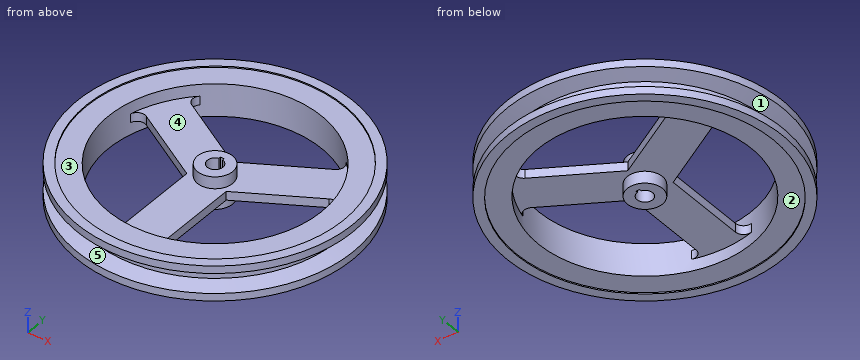
```python
from build123d import *

# Parameters (mm, degrees)
EXTRUDE_1_DEPTH     = 3.5
FILLET_1_R          = 6.5
SKETCH_4_R          = 14
EXTRUDE_2_DEPTH     = 13
CUT_EXTRUDE_1_DEPTH = 13


with BuildPart() as part:
    # 草图2 → 旋转1 (revolve)
    with BuildSketch(Plane(origin=(0, 0, 0), x_dir=(0, 0, -1), z_dir=(1, 0, 0)), mode=Mode.PRIVATE) as revolve_1_sk:
        Polygon((14, 102.5), (14, 110), (8, 110), (5.707749251, 97), (-5.707749251, 97), (-8, 110), (-14, 110), (-14, 102.5), (-13, 102.5), (-13, 85), (13, 85), (13, 102.5), align=None)
    revolve(revolve_1_sk.sketch.rotate(Axis((0, 0, 67.916666667), (0, 0, -1)), 90), axis=Axis((0, 0, 67.916666667), (0, 0, -1)))

    # 草图3 → 凸台-拉伸1 (add, symmetric)
    with BuildSketch(Plane.XY):
        with BuildLine():
            Line((0, 18.186533479), (-64.462425479, 55.403932183))
            ThreePointArc((-64.462425479, 55.403932183), (-73.612159322, 42.5), (-80.212425479, 28.124131963))
            Line((-80.212425479, 28.124131963), (-15.75, -9.09326674))
            Line((-15.75, -9.09326674), (-15.75, -83.528064146))
            ThreePointArc((-15.75, -83.528064146), (0, -85), (15.75, -83.528064146))
            Line((15.75, -83.528064146), (15.75, -9.09326674))
            Line((15.75, -9.09326674), (80.212425479, 28.124131963))
            ThreePointArc((80.212425479, 28.124131963), (73.612159322, 42.5), (64.462425479, 55.403932183))
            Line((64.462425479, 55.403932183), (0, 18.186533479))
        make_face()
    extrude(amount=EXTRUDE_1_DEPTH, both=True)

    # 圆角1
    fillet_1_edges = [part.edges().sort_by_distance(p)[0] for p in [
        (64.462425479, 55.403932183, 0),
        (-64.462425479, 55.403932183, 0),
        (-80.212425479, 28.124131963, 0),
        (-15.75, -83.528064146, 0),
        (15.75, -83.528064146, 0),
        (80.212425479, 28.124131963, 0),
    ]]
    fillet(fillet_1_edges, radius=FILLET_1_R)

    # 草图4 → 凸台-拉伸2 (add, symmetric)
    with BuildSketch(Plane.XY):
        with Locations(Location((0, 0, 0), (0, 0, 180))):
            Circle(SKETCH_4_R)
    extrude(amount=EXTRUDE_2_DEPTH, both=True)

    # 草图5 → 切除-拉伸1 (cut, symmetric)
    with BuildSketch(Plane.XY):
        with BuildLine():
            Line((-1.5, 6.06733055), (-1.5, 7.75))
            Line((-1.5, 7.75), (1.5, 7.75))
            Line((1.5, 7.75), (1.5, 6.06733055))
            ThreePointArc((1.5, 6.06733055), (0, -6.25), (-1.5, 6.06733055))
        make_face()
    extrude(amount=CUT_EXTRUDE_1_DEPTH, both=True, mode=Mode.SUBTRACT)


solid = part.part
```
Model file for the job. Use its own axes, mm. Face numbers are marked on the shaded views. A direction names the side the tool comes from. Round coordinates to 2 decimals unless told otherwise and drop trailing zeros. Put each result on its own line as item: value. Start each with the question number.
Item 1: Drill centre lines: line 1 along Y through (x, z) = (18.5, 0.75); line 2 along X through (y, z) = (3, 11); line 3 along Y through (x, z) = (0, -13.6). Where is each one in solid material? Low to high.
Item 2: Mould opens along Y. For the marked faces 4 and 5 say: released by +Y, released by -Y, zero draft, split by the parting line, or undercut.
Item 3: 3-axis set-ups, long thin cutter, end or side, ignore diameter. For the marked faces 1, 2 and 3: which of +Z, -Z, +X, -X, +Y, -Y reach the whole face in a straight line?
Item 4: Cut at A-A (y = 0). Give the number of separate pieces and of enclosed holes in the cut face, then the cut area to 3 significant figures.
Item 5: Drop flat-ended pins along their axis: P1, Ø10, axis at x = -53, y = 18.5, coming from the +Z side; P2, Ø14, axis at x = -6.5, y = 2, coming from the +Z side; P3, Ø12, axis at x = 81, z = 3, coming from the -Y side; P4, Ø8, axis at x = -83, y = -79, coming from the +Z side. Give the stop position or say it passes through.
Answer block:
1. line 1: -95.22 to -80.59, -7.51 to 28.87, 82.96 to 95.22
1. line 2: -109.96 to -84.95, -13.67 to -5.48, 5.48 to 13.67, 84.95 to 109.96
1. line 3: -110 to -102.5, 102.5 to 110
2. face 4: undercut
2. face 5: split by the parting line
3. face 1: none
3. face 2: -Z
3. face 3: +Z
4. separate pieces: 4
4. enclosed holes: 0
4. area: 1,620 mm2
5. P1: z = 3.5
5. P2: z = 13
5. P3: y = -77.88
5. P4: through
